Verification items for this drawing (mm, ordinates from the low corner). A direction names the side the tool comes from. Give positions to 0.01 mm unless a question says otherwise; leave off trailing zeros. Order: outer loops, then holes, each group sorted by start corner. A loop starts at its lowest first (then second) coordinate and runs counter-clockwise, first axis right, second up.
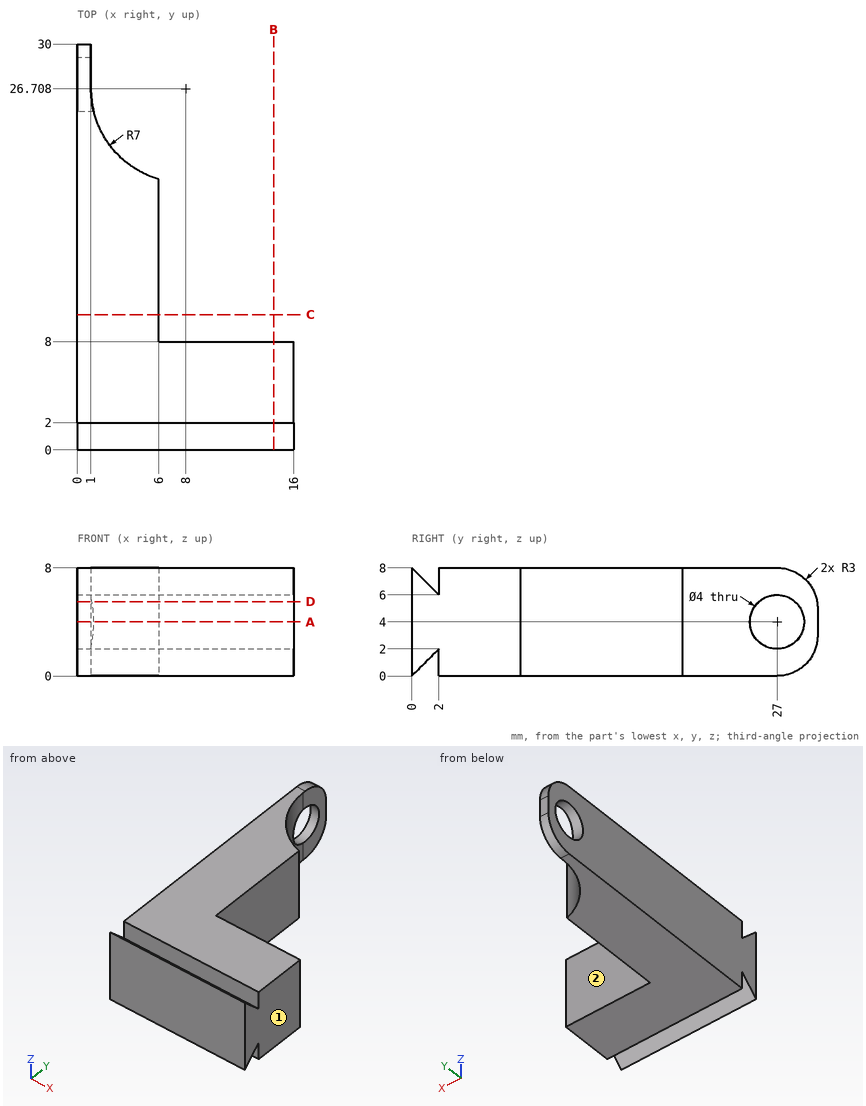
Q1. Cross-section at D-D, the plane z = 5.5. Record the boundary of the cut face in (x, y), and give its area (3 significant figures).
Q2. Thickness scan on L1, parallel to Y at x = 0.6, z = 4; L2, parallel to Z at x = 0.85, y = 27; L3, parallel to Y at x = 9.75, z = 4.5. Record the ranges inside material, lowest first.
Q3. Gauge pin test, flat ends, axial feed: P1, Ø2.5, axis at y = 28, z = 5.5, coming from the +X side; P2, Ø4, axis at y = 12.5, z = 5.5, coming from the +X side; P3, Ø3.5, axis at y = 27, z = 4, coming from the +X side; P4, Ø1.5, axis at x = 6, z = 5, coming from the +Y side. Record the tip position at first contact, or that the pin passes through.
Q4. Cross-section at C-C, the plane y = 10. Record the boundary of the cut face in (x, z).
Q5. Cross-section at A-A, the plane z = 4. Record the boundary of the cut face in (x, y).
Q6. Access from +Z, -Z, +X, -X, +Y, -Y to the whole of each face (thin tool, end or side, straight path). Record for the marked faces 1 and 2.
Q7. Cross-section at B-B, the plane x = 14.5. Record the boundary of the cut face in (y, z), and give its area (3 significant figures).
Answers follow:
1. outline: (0, 0) - (16, 0) - (16, 8) - (6, 8) - (6, 20) arc R7 cw to (1.08, 25.68) - (0, 25.68) - close; (0, 28.32) - (1, 28.32) - (1, 29.96) - (0, 29.96) - close
1. area: 216 mm2
2. L1: y = 0 to 25, 29 to 30
2. L2: z = 0 to 2, 6 to 8
2. L3: y = 0 to 8
3. P1: stops at x = 1
3. P2: stops at x = 6
3. P3: passes through
3. P4: stops at y = 20.27
4. outline: (0, 0) - (6, 0) - (6, 8) - (0, 8) - close
5. outline: (0, 0) - (16, 0) - (16, 8) - (6, 8) - (6, 20) arc R7 cw to (1.21, 25) - (0, 25) - close; (0, 29) - (1, 29) - (1, 30) - (0, 30) - close
6. face 1: +Z, -Z, +X, +Y, -Y
6. face 2: +Z, -Z, +X, +Y
7. outline: (0, 0) - (2, 2) - (2, 0) - (8, 0) - (8, 8) - (2, 8) - (2, 6) - (0, 8) - close
7. area: 60.0 mm2
